Can you work these out from the model? Positions are in its coordinate system, mm. A direction names the side the tool comes from. Coordinates: 2 decimals unless noted, no trailing zeros. Order: outer loops, then holes, each group sorted by start corner. A loop starts at its lowest first (then second) coordinate and runs counter-clockwise, first axis right, second up. Notation, with made-up numbers: (79, -31) -> (117, -31) arc R20 ccw to (117, -25) -> close; hole circle Ø9 at (82.25, 72.25). An arc over 180 degrees is marked (long way). Answer in a Markdown table with one row per item. Add a question column.
1. Imagine slicing it at C-C on z = 16. Write out the boundary of the cut face in (x, y).
2. Imagine slicing it at B-B on x = 25. Write out the boundary of the cut face in (y, z), plus the area to 4 significant figures.
3. If I drill on line 1 along Z through (x, y) = (35, 46); line 2 along Y through (x, z) = (1.5, 15.5), over which ranges is the centre line in solid material (lowest first)? Write a range as [from, to].
4. We'd pull the mould along X, two halves only. Please class faces 5 (the face through (60, 28, 62)), 6 (the face through (12, 6, 37)), 7 (the face through (0, 36, 40)), 8 (the face through (41, 0, 22)): pulls with the +X half, pulls with the -X half, needs draft (parallel to the pull), parting line crosses it, or undercut.
5. Imagine slicing it at D-D on x = 1.5. Write out the boundary of the cut face in (y, z), plus the area to 3 significant figures.
6. Will these pins go through, and if not, where does the flat tip stop? pin 1 (15 mm diameter, centred on y = 14, z = 23, fed in from -X); pin 2 (8 mm diameter, centred on y = 46, z = 71.5, fed in from +X); pin 3 (8 mm diameter, centred on x = -5, y = 24.5, fed in from -Z).
7. On a 3-axis mill with a long thin cutter (end or side, diameter ignored), from which of +Z, -Z, +X, -X, +Y, -Y can I reach the whole of each face in a straight line? I mean faces 1 (the face through (-5, 30, 65)), 2 (the face through (50, 25, 63)), 3 (the face through (40, 45, 17)), 4 (the face through (50, 36, 40)). Say none if no direction works.
8. Imagine slicing it at A-A on y = 28.5. Write out the boundary of the cut face in (x, z).
Autodesk Fusion 360 part; units mm, degrees
sketch "Sketch1" plane through (0, 0, 0) normal (0, 0, 1) x (1, 0, 0) in component "Chair Brutaliste"
  line L0 (0, 0) -> (10, 0)
  line L1 (10, 0) -> (10, 10)
  line L2 (10, 10) -> (0, 10)
  line L3 (0, 10) -> (0, 0)
  line L4 (0, 0) -> (50, 0) construction
  line L5 (50, 0) -> (50, 50) construction
  line L6 (50, 50) -> (0, 50) construction
  line L7 (50, 0) -> (40, 0)
  line L8 (40, 0) -> (40, 10)
  line L9 (40, 10) -> (50, 10)
  line L10 (50, 10) -> (50, 0)
  line L11 (50, 50) -> (40, 50)
  line L12 (40, 50) -> (40, 40)
  line L13 (40, 40) -> (50, 40)
  line L14 (50, 40) -> (50, 50)
  line L15 (0, 50) -> (10, 50)
  line L16 (10, 50) -> (10, 40)
  line L17 (10, 40) -> (0, 40)
  line L18 (0, 40) -> (0, 50)
  dimension "d1" = 10
  dimension "d2" = 50
extrude "Extrude1" add sketch "Sketch1" along normal blind 40 makes body 1 at (3.3333, 50, 13.3333) makes body 2 at (0, 6.6667, 13.3333) makes body 3 at (50, 43.3333, 13.3333) makes body 4 at (43.3333, 10, 13.3333) in component "Chair Brutaliste"
sketch "Sketch2" plane through (0, 0, 40) normal (0, 0, 1) x (-1, 0, 0) in component "Chair Brutaliste"
  line L0 (-50, -10) -> (-40, -10)
  line L1 (-40, -10) -> (-40, 0)
  line L2 (-40, 0) -> (-50, 0)
  line L3 (-50, 0) -> (-50, -10)
  line L4 (-50, -50) -> (0, -50)
  line L5 (0, -50) -> (0, 0)
  line L6 (0, 0) -> (-50, 0)
  line L7 (-50, 0) -> (-50, -50)
extrude "Extrude2" add sketch "Sketch2" along normal blind 10 bodies 1 2 3 4 in component "Chair Brutaliste"
sketch "Sketch3" plane through (50, 0, 0) normal (1, 0, 0) x (0, 1, 0) in component "Chair Brutaliste"
  line L0 (40, 0) -> (50, 0)
  line L1 (50, 0) -> (50, 50)
  line L2 (50, 50) -> (0, 50)
  line L3 (0, 50) -> (0, 0)
  line L4 (0, 0) -> (10, 0)
  line L5 (10, 0) -> (10, 40)
  line L6 (10, 40) -> (40, 40)
  line L7 (40, 40) -> (40, 0)
  line L8 (50, 50) -> (40, 50)
  line L9 (40, 50) -> (40, 95)
  line L10 (40, 95) -> (50, 95)
  line L11 (50, 95) -> (50, 50)
  dimension "d8" = 10
  dimension "d9" = 45
extrude "Extrude3" add sketch "Sketch3" against normal up to surface (50 mm away) contours L2 L8 L9 L10 L11 bodies 1 in component "Chair Brutaliste"
sketch "Sketch4" plane through (0, 40, 0) normal (0, -1, 0) x (1, 0, 0) in component "Chair Brutaliste"
  line L0 (0, 95) -> (0, 50)
  line L1 (0, 50) -> (50, 50)
  line L2 (50, 50) -> (50, 95)
  line L3 (50, 95) -> (0, 95)
  line L4 (10, 60) -> (40, 60)
  line L5 (40, 60) -> (40, 85)
  line L6 (40, 85) -> (10, 85)
  line L7 (10, 85) -> (10, 60)
  dimension "d13" = -10
extrude "Extrude4" cut sketch "Sketch4" against normal up to surface (10 mm away) contours L4 L5 L6 L7 bodies 1 in component "Chair Brutaliste"
chamfer "Chamfer2" distance 5 angle 45 8 edges at (10, 45, 40) (10, 5, 40) (40, 45, 40) (40, 5, 40) (5, 40, 40) (5, 10, 40) (45, 40, 40) (45, 10, 40) on bodies 1 in component "Chair Brutaliste"
chamfer "Chamfer3" distance 3 angle 45 4 edges at (40, 45, 85) (10, 45, 85) (10, 45, 60) (40, 45, 60) on bodies 1 in component "Chair Brutaliste"
chamfer "Chamfer4" distance 6 angle 45 2 edges at (50, 45, 95) (0, 45, 95) on bodies 1 in component "Chair Brutaliste"
sketch "Sketch5" plane through (50, 0, 0) normal (1, 0, 0) x (0, 1, 0) in component "Chair Brutaliste"
  line L0 (50, 89) -> (40, 89)
  line L1 (40, 89) -> (40, 50)
  line L2 (40, 50) -> (0, 50)
  line L3 (0, 50) -> (0, 0)
  line L4 (0, 0) -> (10, 0)
  line L5 (10, 0) -> (10, 35)
  line L6 (10, 35) -> (15, 40)
  line L7 (15, 40) -> (35, 40)
  line L8 (35, 40) -> (40, 35)
  line L9 (40, 35) -> (40, 0)
  line L10 (40, 0) -> (50, 0)
  line L11 (50, 0) -> (50, 89)
  line L12 (40, 50) -> (40, 60) construction
  line L13 (40, 60) -> (40, 65)
  line L14 (40, 60) -> (50, 60)
  line L15 (40, 65) -> (50, 65)
  line L16 (50, 60) -> (50, 65)
  dimension "d19" = 5
  dimension "d20" = 10
extrude "Extrude5" add sketch "Sketch5" along normal blind 10 contours L1 L11 L13 L14 L15 L16 bodies 1 in component "Chair Brutaliste"
sketch "Sketch6" plane through (0, 40, 0) normal (0, -1, 0) x (1, 0, 0) in component "Chair Brutaliste"
  line L0 (13, 85) -> (37, 85)
  line L1 (37, 85) -> (40, 82)
  line L2 (40, 82) -> (40, 63)
  line L3 (40, 63) -> (37, 60)
  line L4 (37, 60) -> (13, 60)
  line L5 (13, 60) -> (10, 63)
  line L6 (10, 63) -> (10, 82)
  line L7 (10, 82) -> (13, 85)
  line L8 (6, 95) -> (0, 89)
  line L9 (0, 89) -> (0, 50)
  line L10 (0, 50) -> (50, 50)
  line L11 (50, 50) -> (50, 60)
  line L12 (50, 60) -> (60, 60)
  line L13 (60, 60) -> (60, 65)
  line L14 (60, 65) -> (50, 65)
  line L15 (50, 65) -> (50, 89)
  line L16 (50, 89) -> (44, 95)
  line L17 (44, 95) -> (6, 95)
  line L18 (50, 65) -> (50, 60)
extrude "Extrude6" add sketch "Sketch6" along normal blind 30 contours L12 L13 L14 L18 bodies 1 in component "Chair Brutaliste"
ref_plane "WorkPlane1" through (25, 25, 44.5) normal (-1, 0, 0) x (0, -1, 0) in component "Chair Brutaliste"
mirror "Mirror1" about plane through (25, 25, 44.5) normal (-1, 0, 0) of "Extrude5" in component "Chair Brutaliste"
sketch "Sketch7" plane through (0, 40, 0) normal (0, -1, 0) x (1, 0, 0) in component "Chair Brutaliste"
  line L0 (50, 60) -> (50, 65)
  line L1 (50, 65) -> (50, 89)
  line L2 (50, 89) -> (44, 95)
  line L3 (44, 95) -> (6, 95)
  line L4 (6, 95) -> (0, 89)
  line L5 (0, 89) -> (0, 65)
  line L6 (0, 65) -> (-10, 65)
  line L7 (-10, 65) -> (-10, 60)
  line L8 (-10, 60) -> (0, 60)
  line L9 (0, 60) -> (0, 50)
  line L10 (0, 50) -> (50, 50)
  line L11 (13, 85) -> (37, 85)
  line L12 (37, 85) -> (40, 82)
  line L13 (40, 82) -> (40, 63)
  line L14 (40, 63) -> (37, 60)
  line L15 (37, 60) -> (13, 60)
  line L16 (13, 60) -> (10, 63)
  line L17 (10, 63) -> (10, 82)
  line L18 (10, 82) -> (13, 85)
  line L19 (0, 65) -> (0, 60)
  line L20 (50, 50) -> (50, 60)
extrude "Extrude7" add sketch "Sketch7" along normal up to surface (30 mm away) contours L6 L7 L8 L19 bodies 1 in component "Chair Brutaliste"
chamfer "Chamfer6" distance 5 angle 45 1 edges at (25, 0, 50) on bodies 1 in component "Chair Brutaliste"
chamfer "Chamfer7" distance 5 angle 45 2 edges at (60, 50, 62.5) (-10, 50, 62.5) on bodies 1 in component "Chair Brutaliste"
chamfer "Chamfer8" distance 5 angle 45 2 edges at (50, 45, 60) (0, 45, 60) on bodies 1 in component "Chair Brutaliste"
component "Chair Brutaliste" placed x (1, 0, 0) y (0, 1, 0) z (0, 0, 1) at (0, 0, 0)
Answers follow:
| question | item | result |
|---|---|---|
| 1 | outline | (0, 0) -> (10, 0) -> (10, 10) -> (0, 10) -> close; (0, 40) -> (10, 40) -> (10, 50) -> (0, 50) -> close; (40, 0) -> (50, 0) -> (50, 10) -> (40, 10) -> close; (40, 40) -> (50, 40) -> (50, 50) -> (40, 50) -> close |
| 2 | outline | (0, 40) -> (50, 40) -> (50, 60) -> (40, 60) -> (40, 50) -> (5, 50) -> (0, 45) -> close; (40, 85) -> (50, 85) -> (50, 95) -> (40, 95) -> close |
| 2 | area | 687.5 mm² |
| 3 | line 1 | z = [40, 60], [85, 95] |
| 3 | line 2 | y = [0, 10], [40, 50] |
| 4 | face 5 | pulls with the +X half |
| 4 | face 6 | undercut |
| 4 | face 7 | pulls with the -X half |
| 4 | face 8 | needs draft |
| 5 | outline | (0, 0) -> (10, 0) -> (10, 35) -> (15, 40) -> (35, 40) -> (40, 35) -> (40, 0) -> (50, 0) -> (50, 90.5) -> (40, 90.5) -> (40, 50) -> (5, 50) -> (0, 45) -> close |
| 5 | area | 1,720 mm² |
| 6 | pin 1 | stops at x = 0 |
| 6 | pin 2 | stops at x = 50 |
| 6 | pin 3 | stops at z = 60 |
| 7 | face 1 | +Z, -X, +Y, -Y |
| 7 | face 2 | +Z, -Y |
| 7 | face 3 | -Z, +Y, -Y |
| 7 | face 4 | -Z, +X, +Y, -Y |
| 8 | outline | (-10, 60) -> (0, 60) -> (0, 65) -> (-10, 65) -> close; (0, 40) -> (50, 40) -> (50, 50) -> (0, 50) -> close; (50, 60) -> (60, 60) -> (60, 65) -> (50, 65) -> close |
